Study the drawing (mm; zero at the part's minimum x, y, z) and answer. A direction names the side the tool comes from. Round coordinates to 2 decimals unless told otherwise and drop trailing zeros. Loops run counter-clockwise (first coordinate to the right, second up) from the corner with the lowest first, then second, coordinate; pieces in that order, holes last. Notation, with made-up numbers: (32, -39.5) -> (64, -39.5) arc R14 ccw to (64, -25.5) -> close; hole circle Ø6 at (32, 54.5). An arc over 180 degrees is marked (long way). Use one line per item in the form item = value.
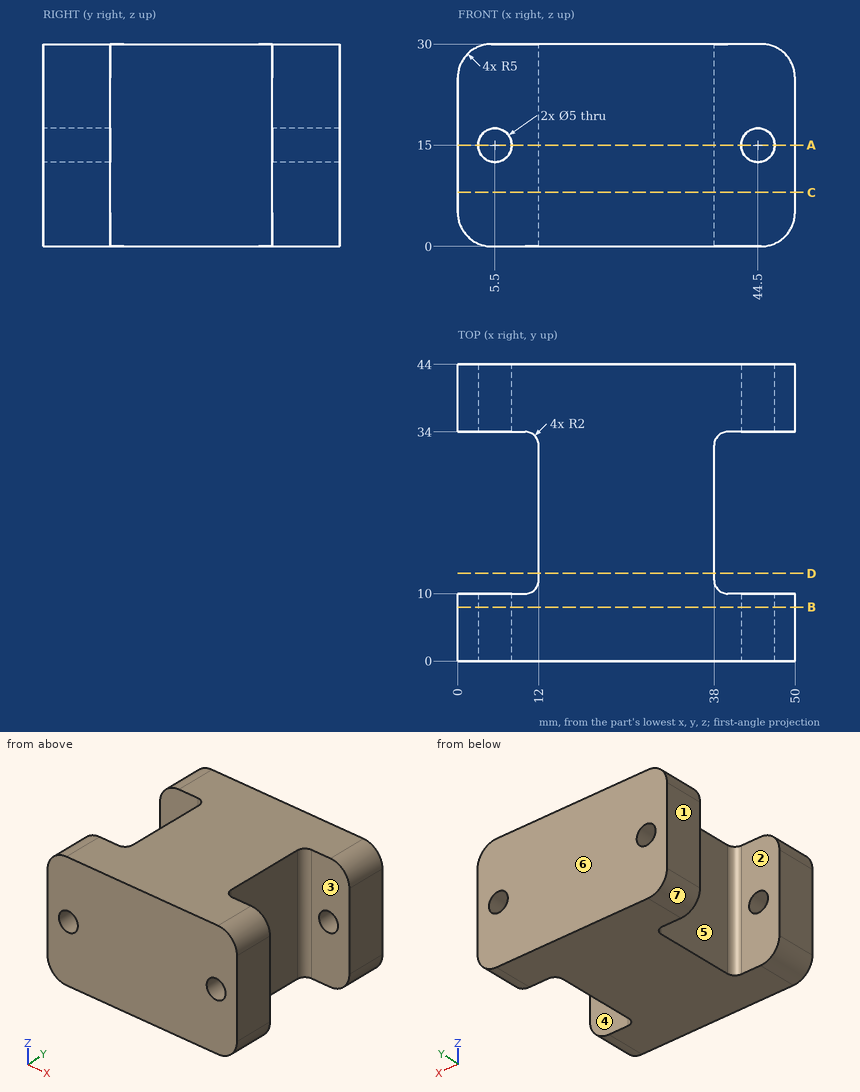
(1) Given P1, Ø10, axis at y = 21, z = 19, coming from the +X side; P2, Ø16, axis at y = 22.5, z = 11.5, coming from the -X side; P3, Ø3, axis at y = 38.5, z = 3, coming from the -X side, each flat-ended and moving along its own axis, determine where each tip first touches the part or whether it passes through.
Completed:
P1 = 38
P2 = 12
P3 = 0.03
(2) Consider L1, parallel to X at y = 6.5, z = 15; L2, parallel to Y at x = 6, z = 25.5; L3, parallel to Z at x = 44.5, y = 39.75. Determine where each line is inside the solid, lowest interval first.
Completed:
L1 = 0 to 3, 8 to 42, 47 to 50
L2 = 0 to 10, 34 to 44
L3 = 0 to 12.5, 17.5 to 30
(3) For a pull along Y with two mould halves and no side action, classify the marked faces 4, 5, 6 and 7 as +Y half, -Y half, draft (parallel to the pull), parting line (faces both ways), or undercut.
Completed:
face_4 = undercut
face_5 = undercut
face_6 = +Y half
face_7 = draft
(4) For the marked faces 1, 2 and 3, determine the directions among +Z, -Z, +X, -X, +Y, -Y from which every point of the face is accessible in a straight line to the end or side of a thin tool.
Completed:
face_1 = +Z, -Z, -X, +Y, -Y
face_2 = +Z, -Z, -X
face_3 = +Z, -Z, +X
(5) Find section A-A, the plane z = 15. State how many separate pieces and enclosed holes the cut face has, then the cut area to 3 significant figures.
Completed:
separate_pieces = 5
enclosed_holes = 0
area = 1,430 mm2
(6) Find section B-B, the plane y = 8. Write down the section's boundary in (x, z), then the cut area to 3 significant figures.
Completed:
outline = (0, 5) arc R5 ccw to (5, 0) -> (45, 0) arc R5 ccw to (50, 5) -> (50, 25) arc R5 ccw to (45, 30) -> (5, 30) arc R5 ccw to (0, 25) -> close; hole circle Ø5 at (5.5, 15); hole circle Ø5 at (44.5, 15)
area = 1,440 mm2
(7) Find section D-D, the plane y = 13. Write down the section's boundary in (x, z), then the cut area to 3 significant figures.
Completed:
outline = (12, 0) -> (38, 0) -> (38, 30) -> (12, 30) -> close
area = 780 mm2
(8) Find section C-C, the plane z = 8. Write down the section's boundary in (x, y).
Completed:
outline = (0, 0) -> (50, 0) -> (50, 10) -> (40, 10) arc R2 cw to (38, 12) -> (38, 32) arc R2 cw to (40, 34) -> (50, 34) -> (50, 44) -> (0, 44) -> (0, 34) -> (10, 34) arc R2 cw to (12, 32) -> (12, 12) arc R2 cw to (10, 10) -> (0, 10) -> close
